```python
from build123d import *

# Parameters (mm, degrees)
ESQUISSE1_R             = 2.25
BOSS_EXTRU_1_DEPTH      = 6
CONG_2_R                = 6
CONG_3_R                = 20
ESQUISSE2_R             = 10.75
BOSS_EXTRU_2_DEPTH      = 4.5
ENL_V_MAT_EXTRU_1_DEPTH = 3


with BuildPart() as part:
    # Esquisse1 → Boss.-Extru.1 (new body)
    with BuildSketch(Plane.XY):
        Polygon((-55, 20), (-27.5, 0), (0, 20), (0, 40), (-55, 40), align=None)
        with Locations((-47.5, 32.5)):
            Circle(ESQUISSE1_R, mode=Mode.SUBTRACT)
        with Locations((-7.5, 32.5)):
            Circle(ESQUISSE1_R, mode=Mode.SUBTRACT)
        with Locations((-27.5, 7.5)):
            Circle(ESQUISSE1_R, mode=Mode.SUBTRACT)
    extrude(amount=BOSS_EXTRU_1_DEPTH)

    # Congé2
    cong_2_edges = [part.edges().sort_by_distance(p)[0] for p in [
        (-55, 40, 3),
        (0, 40, 3),
        (-27.5, 0, 3),
    ]]
    fillet(cong_2_edges, radius=CONG_2_R)

    # Congé3
    cong_3_edges = [part.edges().sort_by_distance(p)[0] for p in [
        (0, 20, 3),
        (-55, 20, 3),
    ]]
    fillet(cong_3_edges, radius=CONG_3_R)

    # Esquisse2 → Boss.-Extru.2 (add)
    with BuildSketch(Plane(origin=(0, 0, 0), x_dir=(-1, 0, 0), z_dir=(0, 0, -1))):
        with Locations(Location((27.5, 27.5, 0), (0, 0, 180))):  # turned: the seam where the file's is
            Circle(ESQUISSE2_R)
    extrude(amount=BOSS_EXTRU_2_DEPTH)

    # Esquisse3 → Enlèvement de matière-Révolution5 (revolve, cut)
    with BuildSketch(Plane(origin=(0, 0, -4.5), x_dir=(-1, 0, 0), z_dir=(0, 0, -1))):
        with BuildLine():
            Line((27.5, 30.25), (27.5, 24.75))
            ThreePointArc((27.5, 24.75), (24.75, 27.5), (27.5, 30.25))
        make_face()
    revolve(axis=Axis((-27.5, 30.25, -4.5), (0, -1, 0)), mode=Mode.SUBTRACT)

    # Esquisse4 → Enlèv. mat.-Extru.1 (cut)
    with BuildSketch(Plane.XY.offset(6)):
        Polygon((-43.169872981, 32.5), (-45.334936491, 36.25), (-49.665063509, 36.25), (-51.830127019, 32.5), (-49.665063509, 28.75), (-45.334936491, 28.75), align=None)
        Polygon((-11.830127019, 32.5), (-9.665063509, 28.75), (-5.334936491, 28.75), (-3.169872981, 32.5), (-5.334936491, 36.25), (-9.665063509, 36.25), align=None)
        Polygon((-23.169872981, 7.5), (-25.334936491, 11.25), (-29.665063509, 11.25), (-31.830127019, 7.5), (-29.665063509, 3.75), (-25.334936491, 3.75), align=None)
    extrude(amount=-ENL_V_MAT_EXTRU_1_DEPTH, mode=Mode.SUBTRACT)


solid = part.part
```
Design review of the part built by this model. Coordinates are the model's own, in mm. A direction names the side the tool comes from. Give positions to 0.01 mm unless a question says otherwise; leave off trailing zeros. Loops run counter-clockwise (first coordinate to the right, second up) from the corner with the lowest first, then second, coordinate; pieces in that order, holes last. Notation, with made-up numbers: (24, 19) -> (79, 19) arc R16 ccw to (79, 50) -> close; hole circle Ø9 at (79, 69.5). An arc over 180 degrees is marked (long way). Write each question's results on one line, items separated by ' | '.
Q1. Take a section at A-A, the plane x = -27.5. Write out the cut boundary in (y, z).
Reply:
outline: (1.42, 0) -> (5.25, 0) -> (5.25, 3) -> (3.75, 3) -> (3.75, 6) -> (1.42, 6) -> close; (9.75, 0) -> (16.75, 0) -> (16.75, -4.5) -> (24.75, -4.5) arc R2.75 cw to (30.25, -4.5) -> (38.25, -4.5) -> (38.25, 0) -> (40, 0) -> (40, 6) -> (11.25, 6) -> (11.25, 3) -> (9.75, 3) -> close
Q2. Take a section at C-C, the plane y = 9. Write out the cut boundary in (x, z) (3 decimals).
Reply:
outline: (-39.875, 0) -> (-29.177, 0) -> (-29.177, 3) -> (-30.964, 3) -> (-30.964, 6) -> (-39.875, 6) -> close; (-25.823, 0) -> (-15.125, 0) -> (-15.125, 6) -> (-24.036, 6) -> (-24.036, 3) -> (-25.823, 3) -> close
Q3. Take a section at B-B, the plane z = 4. Write out the cut boundary in (x, y).
Reply:
outline: (-55, 30.18) arc R20 ccw to (-46.76, 14.01) -> (-31.03, 2.57) arc R6 ccw to (-23.97, 2.57) -> (-8.24, 14.01) arc R20 ccw to (0, 30.18) -> (0, 34) arc R6 ccw to (-6, 40) -> (-49, 40) arc R6 ccw to (-55, 34) -> close; hole (-51.83, 32.5) -> (-49.67, 28.75) -> (-45.33, 28.75) -> (-43.17, 32.5) -> (-45.33, 36.25) -> (-49.67, 36.25) -> close; hole (-31.83, 7.5) -> (-29.67, 3.75) -> (-25.33, 3.75) -> (-23.17, 7.5) -> (-25.33, 11.25) -> (-29.67, 11.25) -> close; hole (-11.83, 32.5) -> (-9.67, 28.75) -> (-5.33, 28.75) -> (-3.17, 32.5) -> (-5.33, 36.25) -> (-9.67, 36.25) -> close
Q4. Wall thickness on L1, parallel to X at y = 32.5, z = 1.15; L2, parallel to Y at x = -47.5, z = 1; L3, parallel to X at y = 35.5, z = 4: over which ranges is each line inside the solid? List them lowest first.
Reply:
L1: x = -55 to -49.75, -45.25 to -9.75, -5.25 to 0 | L2: y = 14.57 to 30.25, 34.75 to 40 | L3: x = -54.81 to -50.1, -44.9 to -10.1, -4.9 to -0.19
Q5. Machinability: for faces 4 (the face through (-7.79, 34.73, 1.48)), 5 (the face through (-8, 28.75, 5)), which of the approach directions +Z, -Z, +X, -X, +Y, -Y give a long, thin tool a straight path to every point of the face, cutting with its end or side? Answer none if there is none.
Reply:
face 4: +Z, -Z | face 5: +Z
Q6. Take a section at D-D, the plane y = 21. Write out the cut boundary in (x, z).
Reply:
outline: (-52.77, 0) -> (-36.06, 0) -> (-36.06, -4.5) -> (-18.94, -4.5) -> (-18.94, 0) -> (-2.23, 0) -> (-2.23, 6) -> (-52.77, 6) -> close
Q7. For pin 1 Ø0.9 at (x, z) = (-27, 4) entering from -Y; pin 2 Ø2 at (x, z) = (-43, 2.5) entering from -Y; pin 3 Ø2.5 at (x, z) = (-6.5, 5) entering from -Y; pin 4 Ø2.5 at (x, y) = (-27.5, 7.5) entering from -Z, all flat-tipped, find the tip position at first contact; note any pin that passes through.
Reply:
pin 1: stops at y = 1.42 | pin 2: stops at y = 10.55 | pin 3: stops at y = 14.38 | pin 4: passes through
Q8. The part is to be moulded in two halves that separate along Y. For faces 1 (the face through (-52.76, 20.99, 3.04)), 2 (the face through (-27, 11.25, 5)), 3 (the face through (-22, 17, 0)), say which applies: +Y half, -Y half, draft (parallel to the pull), parting line (faces both ways), or undercut.
Reply:
face 1: -Y half | face 2: undercut | face 3: draft
